Can you work these out from the model? Positions are in its coordinate system, mm. A direction names the side the tool comes from. Give positions to 0.01 mm unless a question says otherwise; leave off trailing zeros. Loops run counter-clockwise (first coordinate to the right, second up) from the corner with the lowest first, then second, coordinate; pieces in that order, holes last. Notation, with made-up numbers: (20, -15.5) -> (71, -15.5) arc R14 ccw to (71, 3.5) -> close; hole circle Ø1 at (34.25, 0.25). An arc over 180 degrees is marked (long way). Use CSV: the item, a comma, the result in double quotes.
from build123d import *

# Parameters (mm, degrees)
SKICA1_W                 = 16.2
SKICA1_H                 = 11.4
P_IDAT_VYSUNUT_M1_DEPTH  = 7
SKICA2_W                 = 3
SKICA2_H                 = 2.5
ODEBRAT_VYSUNUT_M1_DEPTH = 8
ZAOBLIT5_R               = 1


with BuildPart() as part:
    # Skica1 → Přidat vysunutím1 (new body)
    with BuildSketch(Plane.XY):
        with Locations((8.1, 5.7)):
            Rectangle(SKICA1_W, SKICA1_H)
    extrude(amount=P_IDAT_VYSUNUT_M1_DEPTH)

    # Skica2 → Odebrat vysunutím1 (cut, through all)
    with BuildSketch(Plane.XY.offset(7)):
        with Locations((4.5, 1.25)):
            Rectangle(SKICA2_W, SKICA2_H)
        with Locations((14.7, 1.25)):
            Rectangle(SKICA2_W, SKICA2_H)
    extrude(amount=-ODEBRAT_VYSUNUT_M1_DEPTH, mode=Mode.SUBTRACT)

    # Zaoblit5
    zaoblit5_edges = [part.edges().sort_by_distance(p)[0] for p in [
        (16.2, 6.95, 0),
        (9.6, 0, 0),
        (6, 1.25, 0),
        (3, 1.25, 0),
        (4.5, 2.5, 0),
        (14.7, 2.5, 0),
        (13.2, 1.25, 0),
        (8.1, 11.4, 0),
        (1.5, 0, 0),
        (0, 5.7, 0),
    ]]
    fillet(zaoblit5_edges, radius=ZAOBLIT5_R)


solid = part.part
(1) If I drill on L1, parallel to X at y = 0.5, z = 3.75; L2, parallel to Y at x = 5.75, z = 1; L3, parallel to Z at x = 14, y = 2.75, over which ranges is the centre line in solid material (lowest first)? Write a range as from..to.
Answer sheet:
L1,"x = 0..3, 6..13.2"
L2,"y = 2.5..11.4"
L3,"z = 0.34..7"
(2) Will these pins go through, and if not, where does the flat tip stop? pin 1 Ø2.5 at (x, z) = (15.5, 3) entering from -Y; pin 2 Ø0.8 at (y, z) = (1, 3) entering from +X.
Answer sheet:
pin 1,"stops at y = 2.5"
pin 2,"stops at x = 13.2"
(3) If we section it at D-D, the plane y = 2.75: Write out the boundary of the cut face in (x, z).
Answer sheet:
outline,"(0, 1) arc R1 ccw to (1, 0) -> (2, 0) arc R1 ccw to (2.75, 0.34) -> (6.25, 0.34) arc R1 ccw to (7, 0) -> (12.2, 0) arc R1 ccw to (12.95, 0.34) -> (15.95, 0.34) arc R1 ccw to (16.2, 1) -> (16.2, 7) -> (0, 7) -> close"
(4) If we section it at B-B, the plane z = 2.5: Write out the boundary of the cut face in (x, y).
Answer sheet:
outline,"(0, 0) -> (3, 0) -> (3, 2.5) -> (6, 2.5) -> (6, 0) -> (13.2, 0) -> (13.2, 2.5) -> (16.2, 2.5) -> (16.2, 11.4) -> (0, 11.4) -> close"
(5) Which directions (+Z, -Z, +X, -X, +Y, -Y) give clear straight access to the entire face, cutting with the end or side of a thin tool? Please do faces 4 (the face through (8, 6, 0)), 5 (the face through (12.899, 1.774, 0.285)), 6 (the face through (6.301, 1.774, 0.285)), 7 (the face through (3, 1, 4)), 8 (the face through (13.2, 1, 4)).
Answer sheet:
face 4,"-Z, +X, -X, +Y, -Y"
face 5,"-Z, +X, -Y"
face 6,"-Z, -Y"
face 7,"+Z, -Z, -Y"
face 8,"+Z, -Z, +X, -Y"
(6) We'd pull the mould along X, two halves only. Please class faces 1 (the face through (8.213, 11.115, 0.301)), 2 (the face through (2.699, 1.774, 0.285)), 3 (the face through (16.2, 7, 4)): released by +X, released by -X, zero draft, split by the parting line, or undercut.
Answer sheet:
face 1,"zero draft"
face 2,"undercut"
face 3,"released by +X"
(7) If we section it at C-C, the plane x = 14.5: Write out the boundary of the cut face in (y, z), then the cut area to 3 significant figures.
Answer sheet:
outline,"(2.5, 1) arc R1 ccw to (3.5, 0) -> (10.4, 0) arc R1 ccw to (11.4, 1) -> (11.4, 7) -> (2.5, 7) -> close"
area,"61.9 mm2"
(8) If we section it at A-A, the plane y = 1.5: Write out the boundary of the cut face in (x, z).
Answer sheet:
outline,"(0, 1) arc R1 ccw to (1, 0) -> (2, 0) arc R1 ccw to (3, 1) -> (3, 7) -> (0, 7) -> close; (6, 1) arc R1 ccw to (7, 0) -> (12.2, 0) arc R1 ccw to (13.2, 1) -> (13.2, 7) -> (6, 7) -> close"
